from build123d import *

# Parameters (mm, degrees)
F1_DEPTH = 3.175


with BuildPart() as f1:
    # F0 (on Front) → F1 (new body)
    with BuildSketch(Plane.XZ):
        with BuildLine():
            Line((-232.119275, 112.940714), (-232.119275, 39.1325))
            Line((-232.119275, 39.1325), (250.480725, 39.1325))
            ThreePointArc((250.480725, 39.1325), (131.899672, 94.096964), (2.564945, 112.940714))
            Line((2.564945, 112.940714), (-232.119275, 112.940714))
        make_face()
    extrude(amount=F1_DEPTH)

    # F2: F1 across face


with BuildPart() as f1_1:
    add(f1.part)
    add(f1.part.mirror(Plane(origin=(9.180725, -1.5875, 39.1325), x_dir=(1, 0, 0), z_dir=(0, 0, -1))))


solid = f1_1.part
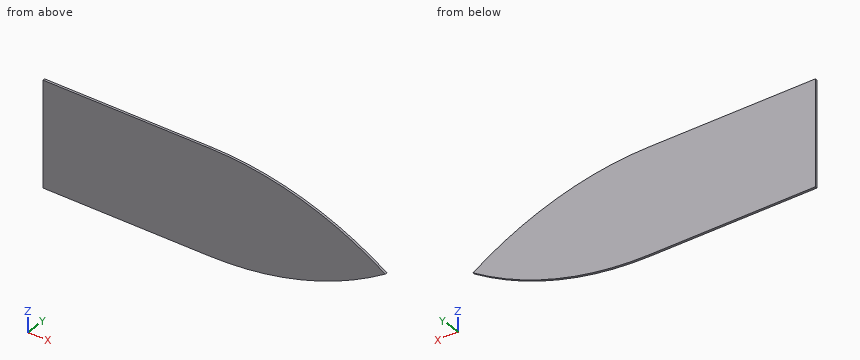
Here's how the part is built. I have some questions about the finished solid (model axes, mm). Round coordinates to 2 decimals unless told otherwise and drop trailing zeros. Write each loop counter-clockwise with the first axis right and the second up, starting at its lowest first coordinate (ties: lowest second). Pieces come first, ordered by that corner, then holes.
1. I need wall thicknesses on L1, parallel to X at y = -2, z = 51; L2, parallel to Z at x = 115.5, y = -0.6; L3, parallel to X at y = -2.05, z = 4.5. Which ranges of each line are inside material? Lowest first, please.
2. Suppose I cut it at B-B (z = 26). List the corners of the cut face in (x, y) for me (3 decimals), and give its area (3 significant figures).
3. Suppose I cut it at A-A (y = -1.15). List the corners of the cut face in (x, z) for me, and give its area (3 significant figures).
4. Suppose I cut it at C-C (x = 184). List the corners of the cut face in (y, z) for me (3 decimals).
Answer sheet:
1. L1: x = -232.12 to 231.29
1. L2: z = -20.38 to 98.65
1. L3: x = -232.12 to 186.9
2. outline: (-232.119, -3.175) - (229.111, -3.175) - (229.111, 0) - (-232.119, 0) - close
2. area: 1,460 mm2
3. outline: (-232.12, -34.68) - (2.56, -34.68) arc R453.27 ccw to (250.48, 39.13) arc R453.27 ccw to (2.56, 112.94) - (-232.12, 112.94) - close
3. area: 59,500 mm2
4. outline: (-3.175, 3.221) - (0, 3.221) - (0, 75.044) - (-3.175, 75.044) - close
